from build123d import *

# Parameters (mm, degrees)
F0_R     = 7.404
F1_DEPTH = 4.5
F3_DEPTH = 4.501
F4_COUNT = 12
F5_R     = 1.1
F6_DEPTH = 4.501


with BuildPart() as f1:
    # F0 (on Front) → F1 (new body)
    with BuildSketch(Plane.XZ):
        Circle(F0_R)
    extrude(amount=F1_DEPTH)

    # F2 (on face) → F3 (cut, through all)
    with BuildSketch(Plane.XZ.offset(4.5)):
        with BuildLine():
            ThreePointArc((-0.5000000047, 5.0005649926), (0, 5.0255), (0.5000000047, 5.0005649926))
            ThreePointArc((0.5000000047, 5.0005649926), (0.7650993145, 6.2330119666), (1.51312227, 7.2477359911))
            ThreePointArc((1.51312227, 7.2477359911), (0, 7.404), (-1.51312227, 7.2477359911))
            ThreePointArc((-1.51312227, 7.2477359911), (-0.7650993145, 6.2330119666), (-0.5000000047, 5.0005649926))
        make_face()
    f3 = extrude(amount=-F3_DEPTH, mode=Mode.SUBTRACT)

    # F4: F3 ×12 about axis
    f4_axis = Axis((0, 0, 0), (0, 1, 0))
    for i in range(1, F4_COUNT):
        add(f3.rotate(f4_axis, i * 360 / F4_COUNT), mode=Mode.SUBTRACT)

    # F5 (on face) → F6 (cut, through all)
    with BuildSketch(Plane.XZ.offset(4.5)):
        Circle(F5_R)
    extrude(amount=-F6_DEPTH, mode=Mode.SUBTRACT)


solid = f1.part
Verification items for the finished model (mm, model axes). A direction names the side the tool comes from. Give positions to 0.01 mm unless a question says otherwise; leave off trailing zeros. Write each loop counter-clockwise with the first axis right and the second up, starting at its lowest first coordinate (ties: lowest second). Pieces come first, ordered by that corner, then holes. Notation, with made-up numbers: M -1.75,62.5 L 15.25,62.5 A17 ccw 15.25,73.5 Z; hole C 13,-33.75 d11. An arc over 180 degrees is marked long. Write item = value, one per line.
(1) Go/stop test with a flat-tipped pin: pin 1 Ø1 at (x, y) = (4, -2.5) entering from -Z. Record where the tip stops, or that it passes through.
Found:
pin_1 = -5.4
(2) Material ranges on line 1 (Z direction, x = 0, y = -3); line 2 (Z direction, x = 4.5, y = -3); line 3 (Z direction, x = -4.75, y = -2.2), recorded low to high.
Found:
line_1 = -5.03 to -1.1, 1.1 to 5.03
line_2 = -5.4 to -3.23, -2.24 to 2.24, 3.23 to 5.4
line_3 = -5.48 to -3.46, -2.16 to 2.16, 3.46 to 5.48
(3) Draft check along X on faces 1 (the face through (1.92, -2.22, 7.15)), 2 (the face through (-5.026, -2.282, -3.794)), 3 (the face through (-4.356, -2.282, 2.507)). Enter one of: released by +X, released by -X, zero draft, split by the parting line, or undercut.
Found:
face_1 = released by +X
face_2 = released by -X
face_3 = undercut
(4) Sectioned sample at A-A (x = 0). Record the cut outline in (y, z).
Found:
outline = M -4.5,-5.03 L 0,-5.03 L 0,-1.1 L -4.5,-1.1 Z; M -4.5,1.1 L 0,1.1 L 0,5.03 L -4.5,5.03 Z
(5) Sectioned sample at B-B (z = 0). Record the cut outline in (x, y), then the cut area to 3 significant figures.
Found:
outline = M -5.03,-4.5 L -1.1,-4.5 L -1.1,0 L -5.03,0 Z; M 1.1,-4.5 L 5.03,-4.5 L 5.03,0 L 1.1,0 Z
area = 35.3 mm2
(6) Access from +Z, -Z, +X, -X, +Y, -Y to the whole of each face (thin tool, end or side, straight path). Record for faces 4 (the face through (-6.249, -2.282, -0.772)), 5 (the face through (-3.794, -2.282, 5.026)), 6 (the face through (2.507, -2.282, 4.356)), 7 (the face through (0.772, -2.282, -6.249)).
Found:
face_4 = -X, +Y, -Y
face_5 = +Z, +Y, -Y
face_6 = +Y, -Y
face_7 = -Z, +Y, -Y
